Autodesk Inventor part; units mm, degrees
ref_plane "YZ Plane" through (0, 0, 0) normal (1, 0, 0) x (0, 1, 0)
ref_plane "XZ Plane" through (0, 0, 0) normal (0, 1, 0) x (-1, 0, 0)
ref_plane "XY Plane" through (0, 0, 0) normal (0, 0, 1) x (1, 0, 0)
sketch "Sketch1" plane through (0, 0, 0) normal (0, 1, 0) x (-1, 0, 0)
  line L0 (-84, 84) -> (84, 84)
  line L1 (84, 84) -> (84, -84)
  line L2 (84, -84) -> (-84, -84)
  line L3 (-84, -84) -> (-84, 84)
  line L4 (-84, 84) -> (84, -84) construction
  line L5 (84, 84) -> (-84, -84) construction
  line L6 (-112.5, 112.5) -> (112.5, 112.5)
  line L7 (112.5, 112.5) -> (112.5, -112.5)
  line L8 (112.5, -112.5) -> (-112.5, -112.5)
  line L9 (-112.5, -112.5) -> (-112.5, 112.5)
  line L10 (-112.5, 112.5) -> (112.5, -112.5) construction
  line L11 (112.5, 112.5) -> (-112.5, -112.5) construction
  point P0 (0, 0)
  dimension "d0" = 168
  dimension "d1" = 168
  dimension "d2" = 225
  dimension "d3" = 225
extrude "Extrusion1" add sketch "Sketch1" along normal blind 2
sketch "Sketch2" plane through (0, 2, 0) normal (0, 1, 0) x (1, 0, 0)
  line L0 (0, 0) -> (-112.5, 0) construction
  line L1 (-112.5, 112.5) -> (-112.5, -112.5)
  circle A0 centre (66.4, -106.5) radius 1.9
  circle A1 centre (66.4, 106.5) radius 1.9
  dimension "d6" = 66.4
  dimension "d7" = 3.8
  dimension "d8" = 106.5
extrude "Extrusion2" cut sketch "Sketch2" against normal blind 2
fillet "Fillet1" radius 5 4 edges at (112.5, 1, -112.5) (112.5, 1, 112.5) (-112.5, 1, -112.5) (-112.5, 1, 112.5)
sketch "Sketch3" plane through (0, 2, 0) normal (0, 1, 0) x (1, 0, 0)
  line L0 (84, 84) -> (84, -84)
  circle A0 centre (80.5, -84) radius 3.5
  line L1 (-84, -84) -> (-84, 84)
  line L2 (0, 0) -> (-84, 0) construction
  line L3 (0, 0) -> (0, -84) construction
  line L4 (84, -84) -> (-84, -84)
  circle A1 centre (-80.5, -84) radius 3.5
  circle A2 centre (80.5, 84) radius 3.5
  circle A3 centre (-80.5, 84) radius 3.5
  point P0 (-84, -84)
  point P1 (-77, -84)
  dimension "d12" = 7
extrude "Extrusion3" cut sketch "Sketch3" against normal blind 2 contours A3 | A1 L4 | A0 L4 | L4 A0 | A2 picked at (-79.4331, -84.8214)
properties part number "Limiter"
The model under review builds one solid part; all positions refer to its coordinate system, in mm. Coordinates: 2 decimals unless noted, no trailing zeros. Write each loop counter-clockwise with the first axis right and the second up, starting at its lowest first coordinate (ties: lowest second). Pieces come first, ordered by that corner, then holes. Notation, with made-up numbers: (21.25, -27) - (56.25, -27) arc R24 cw to (56.25, -15) - close; hole circle Ø8 at (82, 74). An arc over 180 degrees is marked (long way). Answer in a Markdown table with one row per item. Add a question column.
Q1. Consider section C-C on y = 0.6. Give the boundary of the cut face in (x, z).
Q2. Clearance check with a flat-ended pin moving along its axis: pin 1 (12 mm diameter, centred on x = -57, z = -76.5, fed in from -Y). State where the tip first meets the part, or that it passes through.
Q3. Consider section B-B on z = -51. Give the boundary of the cut face in (x, y).
Q4. To check wall thickness, follow line 1 along Z through (x, y) = (66.4, 1.05); line 2 along Z through (x, y) = (-29, 1.8). State the ranges of each line that lie inside material, in increasing order. Write a range as from..to.
Q5. Consider section A-A on x = 4. Give the boundary of the cut face in (y, z).
Answers below:
| question | item | result |
|---|---|---|
| 1 | outline | (-112.5, -107.5) arc R5 ccw to (-107.5, -112.5) - (107.5, -112.5) arc R5 ccw to (112.5, -107.5) - (112.5, 107.5) arc R5 ccw to (107.5, 112.5) - (-107.5, 112.5) arc R5 ccw to (-112.5, 107.5) - close; hole (-84, -84) arc R3.5 ccw to (-77, -84) - (77, -84) arc R3.5 ccw to (84, -84) - (84, 84) arc R3.5 ccw to (77, 84) - (-77, 84) arc R3.5 ccw to (-84, 84) - close; hole circle Ø3.8 at (66.4, -106.5); hole circle Ø3.8 at (66.4, 106.5) |
| 2 | pin 1 | through |
| 3 | outline | (-112.5, 0) - (-84, 0) - (-84, 2) - (-112.5, 2) - close; (84, 0) - (112.5, 0) - (112.5, 2) - (84, 2) - close |
| 4 | line 1 | -112.5..-108.4, -104.6..-84, 84..104.6, 108.4..112.5 |
| 4 | line 2 | -112.5..-84, 84..112.5 |
| 5 | outline | (0, -112.5) - (2, -112.5) - (2, -84) - (0, -84) - close; (0, 84) - (2, 84) - (2, 112.5) - (0, 112.5) - close |
